For this review, take the finished solid that the model builds, in its own axes (mm). Face numbers are marked on the shaded views. Round coordinates to 2 decimals unless told otherwise and drop trailing zeros. Loops run counter-clockwise (first coordinate to the right, second up) from the corner with the lowest first, then second, coordinate; pieces in that order, holes last.
1) Mouldability with a two-part tool opening along Y and no side actions: class the marked faces 1 and 2 as pulls with the +Y half, pulls with the -Y half, needs draft (parallel to the pull), parting line crosses it, or undercut.
2) Take a section at B-B (z = 2.2). State the section outline as (x, y) points.
3) Wall thickness on L1, parallel to Z at x = 32, y = 64; L2, parallel to Y at x = -8, z = 1.65; L3, parallel to Y at x = -68, z = 1.1: over which ranges is each line inside the solid? List them lowest first.
4) Insertion check: pin 1 (1.5 mm diameter, centred on y = -58.5, z = 2.5, fed in from +X); pin 2 (1 mm diameter, centred on x = -42, z = 3, fed in from +Y); pin 3 (1 mm diameter, centred on x = -35, y = -52.5, fed in from -Z). Each pin has a flat end and moves straight along its axis. Give the tip position at first contact, or say it passes through.
5) Take a section at A-A (y = 0). State the section outline as (x, z) points, then the cut area to 3 significant figures.
```python
from build123d import *

# Parameters (mm, degrees)
SKETCH1_R             = 82
SKETCH1_R_2           = 75
BOSS_EXTRUDE1_DEPTH   = 3
SKETCH2_R             = 82
BOSS_EXTRUDE2_DEPTH   = 1
SKETCH4_R             = 5
CUT_EXTRUDE1_DEPTH    = 117.034477635
CIRPATTERN1_COUNT     = 4
M2X0_4_TAPPED_HOLE1_D = 1.6


with BuildPart() as part:
    # Sketch1 → Boss-Extrude1 (new body)
    with BuildSketch(Plane.XY):
        Circle(SKETCH1_R)
        Circle(SKETCH1_R_2, mode=Mode.SUBTRACT)
    extrude(amount=BOSS_EXTRUDE1_DEPTH)

    # Sketch2 → Boss-Extrude2 (add)
    with BuildSketch(Plane.XY.offset(3)):
        Circle(SKETCH2_R)
    extrude(amount=BOSS_EXTRUDE2_DEPTH)

    # Sketch4 → Cut-Extrude1 (cut, through all)
    with BuildSketch(Plane(origin=(0, 0, 0), x_dir=(-1, 0, 0), z_dir=(0, 0, -1))):
        with Locations((0, 83)):
            Circle(SKETCH4_R)
    cut_extrude1 = extrude(amount=-CUT_EXTRUDE1_DEPTH, mode=Mode.SUBTRACT)

    # CirPattern1: Cut-Extrude1 ×4 about axis
    cirpattern1_axis = Axis((0, 0, 0), (0, 0, 1))
    for i in range(1, CIRPATTERN1_COUNT):
        add(cut_extrude1.rotate(cirpattern1_axis, i * 360 / CIRPATTERN1_COUNT), mode=Mode.SUBTRACT)

    # M2x0.4 Tapped Hole1 (through all)
    with Locations(Plane.XY.offset(4)):
        with Locations((55.507882323, 55.507882323)):
            Hole(M2X0_4_TAPPED_HOLE1_D / 2)


solid = part.part
```
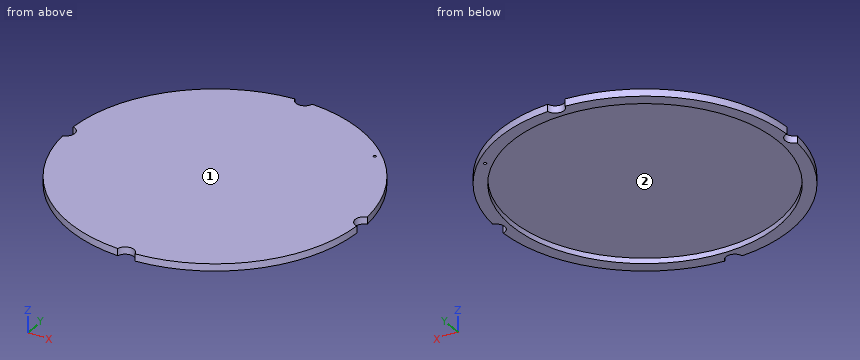
Response:
1. face 1: needs draft
1. face 2: undercut
2. outline: (-81.86, -4.87) arc R82 ccw to (-4.87, -81.86) arc R5 cw to (4.87, -81.86) arc R82 ccw to (81.86, -4.87) arc R5 cw to (81.86, 4.87) arc R82 ccw to (4.87, 81.86) arc R5 cw to (-4.87, 81.86) arc R82 ccw to (-81.86, 4.87) arc R5 cw to start; hole circle Ø150 at (0, 0); hole circle Ø1.6 at (55.51, 55.51)
3. L1: z = 3 to 4
3. L2: y = -81.61 to -74.57, 74.57 to 81.61
3. L3: y = -45.83 to -31.64, 31.64 to 45.83
4. pin 1: stops at x = 58.21
4. pin 2: stops at y = 70.72
4. pin 3: stops at z = 3
5. outline: (-78, 0) - (-75, 0) - (-75, 3) - (75, 3) - (75, 0) - (78, 0) - (78, 4) - (-78, 4) - close
5. area: 174 mm2
